Source: CAD feature listing. Evaluate the final solid. Frame: model axes, mm. Face numbers are marked on the shaded views. Round coordinates to 2 decimals unless told otherwise and drop trailing zeros. Loops run counter-clockwise (first coordinate to the right, second up) from the corner with the lowest first, then second, coordinate; pieces in that order, holes last. Notation, with made-up numbers: M 52,87 L 81,87 A24 ccw 81,99 Z; hole C 34,27.5 d1. An arc over 180 degrees is marked long. Answer as a JSON object with one key per item and string values.
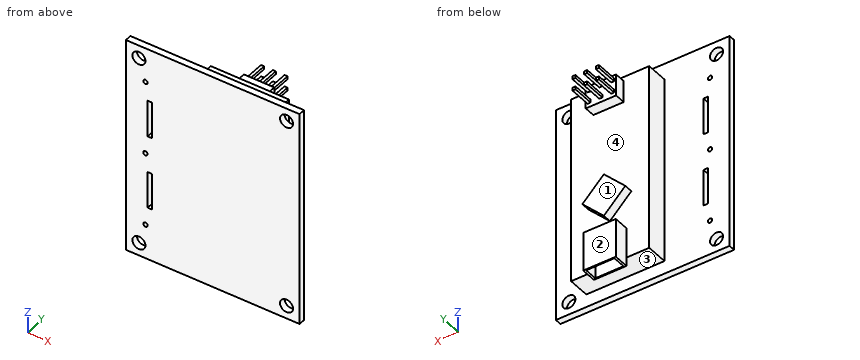
Autodesk Inventor part; units mm, degrees
ref_plane "YZ Plane" through (0, 0, 0) normal (1, 0, 0) x (0, 1, 0)
ref_plane "XZ Plane" through (0, 0, 0) normal (0, 1, 0) x (-1, 0, 0)
ref_plane "XY Plane" through (0, 0, 0) normal (0, 0, 1) x (1, 0, 0)
sketch "Sketch1" plane through (0, 0, 0) normal (0, 1, 0) x (-1, 0, 0)
  line L0 (40, 50) -> (40, 0)
  line L1 (35, 12.25) -> (35, 20.75)
  line L2 (35, 20.75) -> (34, 20.75)
  line L3 (34, 20.75) -> (34, 12.25)
  line L4 (34, 12.25) -> (35, 12.25)
  line L5 (34, 29.25) -> (35, 29.25)
  line L6 (35, 29.25) -> (35, 37.75)
  line L7 (35, 37.75) -> (34, 37.75)
  line L8 (34, 37.75) -> (34, 29.25)
  line L9 (40, 50) -> (0, 50)
  line L10 (0, 0) -> (40, 0)
  line L11 (17.2477, 25) -> (11.4252, 25) construction
  line L12 (0, 0) -> (0, 50)
  circle A0 centre (37, 47) radius 1.5
  circle A1 centre (3, 47) radius 1.5
  circle A2 centre (37, 3) radius 1.5
  circle A3 centre (3, 3) radius 1.5
  point P0 (0, 0)
  point P1 (0, 0)
  point P2 (0, 0)
  point P3 (0, 0)
  point P4 (35.5, 42)
  point P5 (35.5, 25)
  point P6 (35.5, 8)
  dimension "d151" = 8.5
  dimension "d153" = 1
  dimension "d155" = 5
  dimension "d159" = 17
  dimension "d160" = 17
  dimension "d161" = 4.25
  dimension "d162" = 4.25
  dimension "d176" = 4.5
  dimension "d248" = 40
  dimension "d249" = 50
  dimension "d250" = 3
  dimension "d251" = 3
  dimension "d252" = 3
  dimension "d253" = 3
  dimension "d254" = 3
extrude "Extrusion1" add sketch "Sketch1" against normal blind 1.5
hole "Hole1" at (-35.5, 0, 42) at (-35.5, 0, 25) at (-35.5, 0, 8) direction (0, -1, 0) diameter 1 end through all
sketch "Sketch4" plane through (0, 0, 0) normal (0, 1, 0) x (1, 0, 0)
  line L0 (-7, -46.3) -> (-7, -3)
  line L1 (-7, -3) -> (-25, -3)
  line L2 (-25, -3) -> (-25, -46.3)
  line L3 (-25, -46.3) -> (-7, -46.3)
  line L4 (-40, 0) -> (0, 0)
  line L5 (0, 0) -> (0, -50)
  dimension "d189" = 18
  dimension "d255" = 3
  dimension "d256" = 7
  dimension "d257" = 43.3
extrude "Extrusion11" add sketch "Sketch4" along normal blind 5
sketch "Sketch6" plane through (0, 5, 0) normal (0, 1, 0) x (1, 0, 0)
  line L0 (-20.8908, -18.3177) -> (-15.941, -13.368)
  line L1 (-15.941, -13.368) -> (-10.9913, -18.3177)
  line L2 (-10.9913, -18.3177) -> (-15.941, -23.2675)
  line L3 (-15.941, -23.2675) -> (-20.8908, -18.3177)
  point P0 (0, 0)
  dimension "d198" = 7
  dimension "d199" = 7
extrude "Extrusion13" add sketch "Sketch6" along normal blind 2
sketch "Sketch7" plane through (0, 5, 0) normal (0, 1, 0) x (1, 0, 0)
  line L0 (-19.1198, -40.3292) -> (-12.1198, -40.3292)
  line L1 (-12.1198, -40.3292) -> (-12.1198, -45.3292)
  line L2 (-12.1198, -45.3292) -> (-19.1198, -45.3292)
  line L3 (-19.1198, -45.3292) -> (-19.1198, -40.3292)
  point P0 (0, 0)
  dimension "d202" = 7
  dimension "d203" = 5
extrude "Extrusion14" add sketch "Sketch7" along normal blind 2.5
sketch "Sketch8" plane through (0, 7.5, 0) normal (0, 1, 0) x (1, 0, 0)
  line L0 (-18.6618, -41.2282) -> (-17.9618, -41.2282)
  line L1 (-17.9618, -41.2282) -> (-17.9618, -41.9282)
  line L2 (-17.9618, -41.9282) -> (-18.6618, -41.9282)
  line L3 (-18.6618, -41.9282) -> (-18.6618, -41.2282)
  line L4 (-18.6618, -43.9282) -> (-17.9618, -43.9282)
  line L5 (-17.9618, -43.9282) -> (-17.9618, -44.6282)
  line L6 (-17.9618, -44.6282) -> (-18.6618, -44.6282)
  line L7 (-18.6618, -44.6282) -> (-18.6618, -43.9282)
  line L8 (-15.9618, -41.2282) -> (-15.2618, -41.2282)
  line L9 (-15.2618, -41.2282) -> (-15.2618, -41.9282)
  line L10 (-15.2618, -41.9282) -> (-15.9618, -41.9282)
  line L11 (-15.9618, -41.9282) -> (-15.9618, -41.2282)
  line L12 (-15.9618, -43.9282) -> (-15.2618, -43.9282)
  line L13 (-15.2618, -43.9282) -> (-15.2618, -44.6282)
  line L14 (-15.2618, -44.6282) -> (-15.9618, -44.6282)
  line L15 (-15.9618, -44.6282) -> (-15.9618, -43.9282)
  line L16 (-13.2618, -41.2282) -> (-12.5618, -41.2282)
  line L17 (-12.5618, -41.2282) -> (-12.5618, -41.9282)
  line L18 (-12.5618, -41.9282) -> (-13.2618, -41.9282)
  line L19 (-13.2618, -41.9282) -> (-13.2618, -41.2282)
  line L20 (-13.2618, -43.9282) -> (-12.5618, -43.9282)
  line L21 (-12.5618, -43.9282) -> (-12.5618, -44.6282)
  line L22 (-12.5618, -44.6282) -> (-13.2618, -44.6282)
  line L23 (-13.2618, -44.6282) -> (-13.2618, -43.9282)
  point P0 (0, 0)
  dimension "d206" = 0.7
  dimension "d207" = 2
  dimension "d208" = 2
  dimension "d209" = 2
extrude "Extrusion15" add sketch "Sketch8" along normal blind 5
sketch "Sketch9" plane through (-3, 0, 3) normal (0, 0, -1) x (-1, 0, 0)
  line L0 (16.75, 8.5) -> (9.25, 8.5)
  line L1 (9.25, 8.5) -> (9.25, 5)
  line L2 (9.25, 5) -> (16.75, 5)
  line L3 (16.75, 5) -> (16.75, 8.5)
  line L4 (13, 5.7242) -> (13, 7.4058) construction
  line L5 (22, 0) -> (22, 5)
  line L6 (4, 5) -> (22, 5)
  dimension "d213" = 7.5
  dimension "d214" = 3.5
  dimension "d258" = 5.25
extrude "Extrusion16" add sketch "Sketch9" along normal blind 2 and the other way blind 7
sketch "Sketch15" plane through (-3, 0, 1) normal (0, 0, -1) x (-1, 0, 0)
  line L0 (16.25, 8.25) -> (9.75, 8.25)
  line L1 (9.75, 8.25) -> (9.75, 5.25)
  line L2 (9.75, 5.25) -> (16.25, 5.25)
  line L3 (16.25, 5.25) -> (16.25, 8.25)
  line L4 (9.25, 8.5) -> (9.25, 5)
  line L5 (16.75, 8.5) -> (9.25, 8.5)
  point P0 (-3, 0)
  dimension "d242" = 6.5
  dimension "d243" = 3
  dimension "d244" = 0.5
  dimension "d245" = 0.25
extrude "Extrusion20" cut sketch "Sketch15" against normal blind 5
properties part number "Motherboard_dummy" material "ABS Plastic"
Item 1: Section B-B on y = 10. Return the cut outline in (x, z), then the cut area to 3 significant figures.
Answer sheet:
{"outline": "M -18.66,41.23 L -17.96,41.23 L -17.96,41.93 L -18.66,41.93 Z; M -18.66,43.93 L -17.96,43.93 L -17.96,44.63 L -18.66,44.63 Z; M -15.96,41.23 L -15.26,41.23 L -15.26,41.93 L -15.96,41.93 Z; M -15.96,43.93 L -15.26,43.93 L -15.26,44.63 L -15.96,44.63 Z; M -13.26,41.23 L -12.56,41.23 L -12.56,41.93 L -13.26,41.93 Z; M -13.26,43.93 L -12.56,43.93 L -12.56,44.63 L -13.26,44.63 Z", "area": "2.94 mm²"}
Item 2: Pull-direction query (Z, two-part tool) for the marked faces 1, 2, 3 and 4; classes: pulls with the +Z half, pulls with the -Z half, needs draft (parallel to the pull), parting line crosses it, or undercut.
Answer sheet:
{"face 1": "undercut", "face 2": "needs draft", "face 3": "pulls with the -Z half", "face 4": "undercut"}
Item 3: Section C-C on z = 47. Return the cut outline in (x, y), then the cut area to 3 significant figures.
Answer sheet:
{"outline": "M -40,-1.5 L -38.5,-1.5 L -38.5,0 L -40,0 Z; M -35.5,-1.5 L -4.5,-1.5 L -4.5,0 L -35.5,0 Z; M -1.5,-1.5 L 0,-1.5 L 0,0 L -1.5,0 Z", "area": "51.0 mm²"}
Item 4: Section D-D on z = 33. Return the cut outline in (x, y).
Answer sheet:
{"outline": "M -40,-1.5 L -35,-1.5 L -35,0 L -40,0 Z; M -34,-1.5 L 0,-1.5 L 0,0 L -7,0 L -7,5 L -25,5 L -25,0 L -34,0 Z"}
Item 5: Line query: probe 1 along Z at (x, y) = (-37, -0.85); probe 2 along X at (y, z) = (-0.85, 25); probe 3 along Y at (x, z) = (-9, 28). Output: solid intervals per line, ascending. Write a range as from..to.
Answer sheet:
{"probe 1": "z = 0..1.5, 4.5..45.5, 48.5..50", "probe 2": "x = -40..-36, -35..0", "probe 3": "y = -1.5..5"}
Item 6: Section A-A on x = -3. Return the cut outline in (y, z).
Answer sheet:
{"outline": "M -1.5,0 L 0,0 L 0,1.5 L -1.5,1.5 Z; M -1.5,4.5 L 0,4.5 L 0,45.5 L -1.5,45.5 Z; M -1.5,48.5 L 0,48.5 L 0,50 L -1.5,50 Z"}
Item 7: Contact query for flat-ended pins moving along their axis: pin 1 Ø1 at (y, z) = (3.5, 13.5) entering from -X; pin 2 Ø0.6 at (x, y) = (-15.5, 9.5) entering from -Z; pin 3 Ø6 at (x, z) = (-10.5, 37) entering from +Y. Output: stop coordinate, or through.
Answer sheet:
{"pin 1": "stops at x = -25", "pin 2": "stops at z = 41.23", "pin 3": "stops at y = 5"}
